```python
from build123d import *

# Parameters (mm, degrees)
F0_R     = 3
F1_DEPTH = 25
F2_DEPTH = 5
F3_R     = 0.5


with BuildPart() as f1:
    # F0 (on Front) → F1 (new body)
    with BuildSketch(Plane.XZ):
        Circle(F0_R)
    extrude(amount=F1_DEPTH)

    # F0 (on Front) → F2 (join)
    with BuildSketch(Plane.XZ):
        Polygon((-2.886751, -5), (2.886751, -5), (5.773503, 0), (2.886751, 5), (-2.886751, 5), (-5.773503, 0), align=None)
        Circle(F0_R, mode=Mode.SUBTRACT)
        Circle(F0_R)
    extrude(amount=-F2_DEPTH)

    # F3
    f3_edges = [f1.edges().sort_by_distance(p)[0] for p in [
        (-2.886751, 2.5, -5),
        (2.886751, 2.5, -5),
        (0, 0, -5),
        (0, 5, -5),
        (5.773503, 2.5, 0),
        (4.330127, 0, -2.5),
        (4.330127, 5, -2.5),
        (4.330127, 5, 2.5),
        (0, 5, 5),
        (-4.330127, 5, 2.5),
        (-4.330127, 5, -2.5),
        (-5.773503, 2.5, 0),
        (-4.330127, 0, -2.5),
        (-2.886751, 2.5, 5),
        (-4.330127, 0, 2.5),
        (2.886751, 2.5, 5),
        (0, 0, 5),
        (4.330127, 0, 2.5),
    ]]
    fillet(f3_edges, radius=F3_R)


solid = f1.part
```
CAD build for the part. Positions are in the model's coordinates, mm. A direction names the side the tool comes from. Give positions to 0.01 mm unless a question says otherwise; leave off trailing zeros. Write each loop counter-clockwise with the first axis right and the second up, starting at its lowest first coordinate (ties: lowest second). Pieces come first, ordered by that corner, then holes. Notation, with made-up numbers: M 71,85 L 83,85 A27 cw 83,120 Z; hole C 9,49 d1. An arc over 180 degrees is marked long. Return JSON: item names as keys, results as strings. Group by question number.
(1) Flat gauge pins, fed straight in: pin 1 Ø1 at (x, y) = (-1.5, -19.5) entering from +Z; pin 2 Ø6 at (y, z) = (-12, 2.5) entering from +X; pin 3 Ø6 at (y, z) = (-19.5, 2) entering from -X. Where does each tip first touch, or does it go through?
(2) Band-saw the part on B-B (x = 0). Give the cut face in (y, z).
(3) Band-saw the part on A-A (y = 2.5). Give the cut face in (x, z).
(4) 3-axis set-ups, long thin cutter, end or side, ignore diameter. For faces 1 (the face through (4.182, 0.143, 2.456)), 2 (the face through (1, 0, 3)): which of +Z, -Z, +X, -X, +Y, -Y reach the whole face in a straight line?
(5) Drill centre lines: L1, parallel to Y at x = -2.25, z = 2.75; L2, parallel to X at y = -10.25, z = -1.5; L3, parallel to Z at x = -2.75, y = -8.75. Where is each one in solid material? Low to high. Write a range as [from, to].
(6) Band-saw the part on C-C (y = -22.75). Give the cut face in (x, z).
Entries:
{
 "1": {"pin 1": "stops at z = 2.83", "pin 2": "stops at x = 3", "pin 3": "stops at x = -3"},
 "2": {"outline": "M -25,-3 L 0,-3 L 0,-4.5 A0.5 ccw 0.5,-5 L 4.5,-5 A0.5 ccw 5,-4.5 L 5,4.5 A0.5 ccw 4.5,5 L 0.5,5 A0.5 ccw 0,4.5 L 0,3 L -25,3 Z"},
 "3": {"outline": "M -5.63,-0.25 L -3.03,-4.75 A0.5 ccw -2.6,-5 L 2.6,-5 A0.5 ccw 3.03,-4.75 L 5.63,-0.25 A0.5 ccw 5.63,0.25 L 3.03,4.75 A0.5 ccw 2.6,5 L -2.6,5 A0.5 ccw -3.03,4.75 L -5.63,0.25 A0.5 ccw Z"},
 "4": {"face 1": "+Z, +X, -Y", "face 2": "-Y"},
 "5": {"L1": "y = [0, 5]", "L2": "x = [-2.6, 2.6]", "L3": "z = [-1.2, 1.2]"},
 "6": {"outline": "C 0,0 d6"}
}
